from build123d import *

# Parameters (mm, degrees)
EXTRUDE1_DEPTH      = 3
EXTRUDE1_DEPTH_BACK = 3
SKETCH2_W           = 2.5
SKETCH2_H           = 15
SKETCH2_W_2         = 23.75
SKETCH2_H_2         = 3.25
EXTRUDE2_DEPTH      = 1.75
CHAMFER1_SIZE       = 3
CHAMFER1_SIZE2      = 1.732050808
CHAMFER2_SIZE       = 2
CHAMFER2_SIZE2      = 1.738573476
CHAMFER3_SIZE       = 0.5
EXTRUDE3_REACH      = 30.68
SKETCH4_R           = 2
FILLET1_R           = 0.8


# Read off the part's stored shape, not the designer's step: Mirror1
with BuildPart() as part:
    # Sketch1 → Extrude1 (new, two sides: drawn at the far end of the back side and taken through both)
    with BuildSketch(Plane.XY.offset(-EXTRUDE1_DEPTH_BACK)):
        Polygon((0, 0), (0, 20), (-5, 20), (-5, -5), (20, -5), (20, 0), align=None)
    extrude(amount=EXTRUDE1_DEPTH + EXTRUDE1_DEPTH_BACK)

    # Sketch2 → Extrude2 (add)
    with BuildSketch(Plane.XY.offset(3)):
        with Locations((-2.5, 12.5)):
            Rectangle(SKETCH2_W, SKETCH2_H)
        with Locations((8.125, -3.375)):
            Rectangle(SKETCH2_W_2, SKETCH2_H_2)
    extrude(amount=EXTRUDE2_DEPTH)

    # Chamfer1
    chamfer1_edges = [part.edges().sort_by_distance(p)[0] for p in [
        (20, -3.375, 4.75),
        (-3.75, -3.375, 4.75),
    ]]
    chamfer1_side = [part.faces().sort_by_distance(p)[0] for p in [
        (8.125, -3.375, 4.75),
    ]]
    chamfer(chamfer1_edges, length=CHAMFER1_SIZE, length2=CHAMFER1_SIZE2, reference=chamfer1_side[0])

    # Chamfer2
    chamfer2_edges = [part.edges().sort_by_distance(p)[0] for p in [
        (8.125, -5, 4.75),
    ]]
    chamfer2_side = [part.faces().sort_by_distance(p)[0] for p in [
        (8.125, -3.375, 4.75),
    ]]
    chamfer(chamfer2_edges, length=CHAMFER2_SIZE, length2=CHAMFER2_SIZE2, reference=chamfer2_side[0])

    # Chamfer3
    chamfer3_edges = [part.edges().sort_by_distance(p)[0] for p in [
        (-2.5, 20, 4.75),
        (-1.25, 12.5, 4.75),
        (-2.5, 5, 4.75),
        (-3.75, 12.5, 4.75),
    ]]
    chamfer(chamfer3_edges, length=CHAMFER3_SIZE)

    # Mirror1: part across plane


with BuildPart() as part_1:
    add(part.part)
    add(part.part.mirror(Plane.XY))

    # Sketch4 → Extrude3 (cut, up to next)
    with BuildSketch(Plane(origin=(0, 0, 0), x_dir=(1, 0, 0), z_dir=(0, 1, 0)), mode=Mode.PRIVATE) as extrude3_sk1:
        with Locations(Location((13, 0, 0), (0, 0, 270))):
            Circle(SKETCH4_R)
    extrude3_tool1 = extrude(extrude3_sk1.sketch, amount=-EXTRUDE3_REACH, mode=Mode.PRIVATE) & part_1.part
    extrude3 = extrude3_tool1.solids().sort_by_distance((13, 0, 0))[0]
    add(extrude3, mode=Mode.SUBTRACT)

    # Mirror2: Extrude3 across plane
    add(extrude3.mirror(Plane(origin=(0, 0, 0), x_dir=(0, 0, 1), z_dir=(0.7071067811865476, -0.7071067811865475, 0))), mode=Mode.SUBTRACT)

    # Fillet1
    fillet1_edges = [part_1.edges().sort_by_distance(p)[0] for p in [
        (-5, 20, 0),
        (20, -5, 0),
        (20, 0, 0),
        (0, 20, 0),
    ]]
    fillet(fillet1_edges, radius=FILLET1_R)


solid = part_1.part
Source: CAD feature listing. Evaluate the final solid. Frame: model axes, mm. A direction names the side the tool comes from. Give positions to 0.01 mm unless a question says otherwise; leave off trailing zeros. Write each loop counter-clockwise with the first axis right and the second up, starting at its lowest first coordinate (ties: lowest second). Pieces come first, ordered by that corner, then holes. Notation, with made-up numbers: M 69.5,-17 L 94.5,-17 A16 cw 94.5,-3 Z; hole C -0.75,63.5 d11. An arc over 180 degrees is marked long. Return JSON: item names as keys, results as strings. Group by question number.
1) Material intervals for line 1 along Y through (x, z) = (-3.1, 0); line 2 along X through (y, z) = (6.75, 0), sorted ascending. Write a range as [from, to].
2) Cut plane A-A, the plane z = 0. Output: boundary loops of the cut face in (x, y), plus the area to 3 significant figures.
3) Cut plane B-B, the plane y = 13. Output: boundary loops of the cut face in (x, z).
4) Cut plane D-D, the plane x = 5.5. Output: boundary loops of the cut face in (y, z), plus the area to 3 significant figures.
5) Set-up query: faces 5 (the face through (-1.25, 12, -4)), 6 (the face through (-2.6, -3.03, -3.68)), 7 (the face through (-3, 5, -4)), 8 (the face through (0, 9, 0)). Return all of +Z, -Z, +X, -X, +Y, -Y with unobstructed straight access to the full face (end or side cutting, diameter ignored); none if empty.
6) Pin query (flat end, axial travel): P1, Ø3, axis at x = 10, z = 0, coming from the +Y side; P2, Ø2, axis at y = 16.5, z = -1.5, coming from the +X side; P3, Ø1.9, axis at x = 8.5, z = -4, coming from the +Y side. Return the tip coordinate at first contact, or that it passes through.
7) Cut plane C-C, the plane x = 13. Output: boundary loops of the cut face in (y, z).
8) Pull-direction query (Y, two-part tool) for faces 1 (the face through (-3, 5, 4)), 2 (the face through (7.82, -4.01, -3.87)), 3 (the face through (15, -2, 0)), 4 (the face through (-2, 15, 0)); classes: pulls with the +Y half, pulls with the -Y half, needs draft (parallel to the pull), parting line crosses it, or undercut.
Recorded:
{
 "1": {"line 1": "y = [-5, 11], [15, 20]", "line 2": "x = [-5, 0]"},
 "2": {"outline": "M -5,-5 L 11,-5 L 11,0 L 0,0 L 0,11 L -5,11 Z; M -5,15 L 0,15 L 0,19.2 A0.8 ccw -0.8,20 L -4.2,20 A0.8 ccw -5,19.2 Z; M 15,-5 L 19.2,-5 A0.8 ccw 20,-4.2 L 20,-0.8 A0.8 ccw 19.2,0 L 15,0 Z", "area": "184 mm²"},
 "3": {"outline": "M -5,-3 L -3.75,-3 L -3.75,-4.25 L -3.25,-4.75 L -1.75,-4.75 L -1.25,-4.25 L -1.25,-3 L 0,-3 L 0,-2 L -5,-2 Z; M -5,2 L 0,2 L 0,3 L -1.25,3 L -1.25,4.25 L -1.75,4.75 L -3.25,4.75 L -3.75,4.25 L -3.75,3 L -5,3 Z"},
 "4": {"outline": "M -5,-3.01 L -3,-4.75 L -1.75,-4.75 L -1.75,-3 L 0,-3 L 0,3 L -1.75,3 L -1.75,4.75 L -3,4.75 L -5,3.01 Z", "area": "37.9 mm²"},
 "5": {"face 5": "-Z, +X, +Y", "face 6": "-Z, -X, -Y", "face 7": "-Z, +X, -X", "face 8": "+Z, -Z, +X, +Y"},
 "6": {"P1": "stops at y = 0", "P2": "stops at x = 0", "P3": "stops at y = -1.75"},
 "7": {"outline": "M -5,-3.01 L -3,-4.75 L -1.75,-4.75 L -1.75,-3 L 0,-3 L 0,-2 L -5,-2 Z; M -5,2 L 0,2 L 0,3 L -1.75,3 L -1.75,4.75 L -3,4.75 L -5,3.01 Z"},
 "8": {"face 1": "undercut", "face 2": "pulls with the -Y half", "face 3": "needs draft", "face 4": "undercut"}
}
